Answer from the drawing. Dimensions are ordinates in mm from the lowest x, y and z of the part. A direction names the side the tool comes from. Coordinates: 2 decimals unless noted, no trailing zeros. Order: outer loops, then holes, each group sorted by start corner. A loop starts at its lowest first (then second) coordinate and runs counter-clockwise, first axis right, second up. Notation, with made-up numbers: M 74.25,-18 L 131.25,-18 A20 ccw 131.25,-11 Z; hole C -6.5,28.5 d11. An arc over 180 degrees is marked long. Use a Markdown table: item, result.
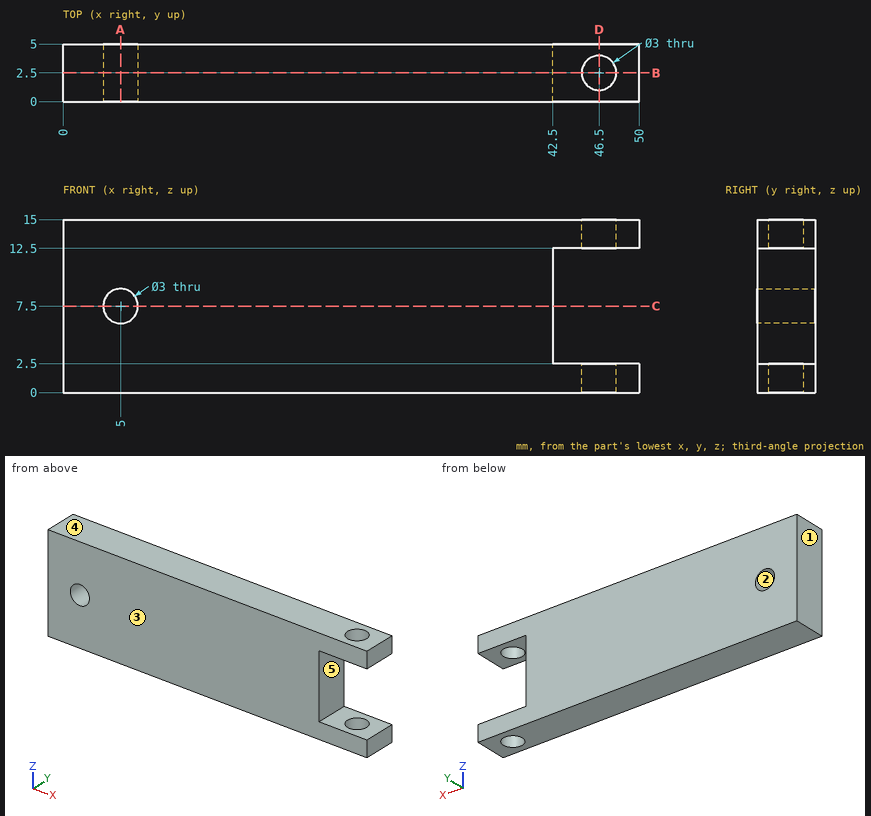
(1) A cutting plane is placed at B-B (y = 2.5). Determine the outline of the cut face in (x, z).
Conclusion:
| item | result |
|---|---|
| outline | M 0,0 L 45,0 L 45,2.5 L 42.5,2.5 L 42.5,12.5 L 45,12.5 L 45,15 L 0,15 Z; M 48,0 L 50,0 L 50,2.5 L 48,2.5 Z; M 48,12.5 L 50,12.5 L 50,15 L 48,15 Z; hole C 5,7.5 d3 |
(2) Given P1, Ø2.5, axis at x = 5, z = 7.5, coming from the +Y side; P2, Ø2.5, axis at y = 2, z = 7, coming from the +X side, each flat-ended and moving along its own axis, determine where each tip first touches the part or whether it passes through.
Conclusion:
| item | result |
|---|---|
| P1 | through |
| P2 | x = 42.5 |
(3) Straight lines are drawn through the part: L1, parallel to X at y = 2.5, z = 14.3; L2, parallel to Y at x = 46.5, z = 13.7; L3, parallel to X at y = 2.2, z = 7.5. For each, find the intervals that lie inside material, in ascending order.
Conclusion:
| item | result |
|---|---|
| L1 | 0 to 45, 48 to 50 |
| L2 | 0 to 1, 4 to 5 |
| L3 | 0 to 3.5, 6.5 to 42.5 |
(4) A cutting plane is placed at D-D (x = 46.5). Determine the outline of the cut face in (y, z), then the cut area to 3 significant figures.
Conclusion:
| item | result |
|---|---|
| outline | M 0,0 L 1,0 L 1,2.5 L 0,2.5 Z; M 0,12.5 L 1,12.5 L 1,15 L 0,15 Z; M 4,0 L 5,0 L 5,2.5 L 4,2.5 Z; M 4,12.5 L 5,12.5 L 5,15 L 4,15 Z |
| area | 10.0 mm2 |
(5) A cutting plane is placed at A-A (x = 5). Determine the outline of the cut face in (y, z), then the cut area to 3 significant figures.
Conclusion:
| item | result |
|---|---|
| outline | M 0,0 L 5,0 L 5,6 L 0,6 Z; M 0,9 L 5,9 L 5,15 L 0,15 Z |
| area | 60.0 mm2 |
(6) Which of the six approach directions +Z, -Z, +X, -X, +Y, -Y give full straight-line access (tool end or side, diameter ignored) to the marked faces 4 and 5?
Conclusion:
| item | result |
|---|---|
| face 4 | +Z, +X, -X, +Y, -Y |
| face 5 | +X, +Y, -Y |
(7) A cutting plane is placed at C-C (z = 7.5). Determine the outline of the cut face in (x, y).
Conclusion:
| item | result |
|---|---|
| outline | M 0,0 L 3.5,0 L 3.5,5 L 0,5 Z; M 6.5,0 L 42.5,0 L 42.5,5 L 6.5,5 Z |
(8) Determine the mould class of the marked faces 1, 2 and 3 for opening direction X: pulls with the +X half, pulls with the -X half, needs draft (parallel to the pull), parting line crosses it, or undercut.
Conclusion:
| item | result |
|---|---|
| face 1 | pulls with the -X half |
| face 2 | undercut |
| face 3 | needs draft |
